Can you work these out from the model? Positions are in its coordinate system, mm. A direction names the side the tool comes from. Give positions to 0.01 mm unless a question says otherwise; leave off trailing zeros. Loops run counter-clockwise (first coordinate to the right, second up) from the corner with the lowest first, then second, coordinate; pieces in that order, holes last. Notation, with made-up numbers: (44.5, 36) - (67.5, 36) arc R19 cw to (67.5, 69) - close; hole circle Ø3 at (71.25, 80). An arc over 180 degrees is marked (long way). Answer as a JSON object with one key per item and string values. Group by question number.
Item 1: Which directions (+Z, -Z, +X, -X, +Y, -Y) give clear straight access to the entire face, cutting with the end or side of a thin tool? Please do faces 4 (the flat face through (0, -20, -2)), 5 (the flat face through (-1, 6, 0)), 6 (the cylindrical face through (1.46, -1.61, 6.95)).
Item 2: Please list where these lines run through material, in increasing order: L1, parallel to Z at x = 0.75, y = -15; L2, parallel to X at y = 23.5, z = 2.25; L3, parallel to Y at x = 0.25, z = -0.5.
Item 3: Will these pins go through, and if not, where does the flat tip stop? pin 1 (0.5 mm diameter, centred on x = 1, z = -0.5, fed in from +Y); pin 2 (1.5 mm diameter, centred on x = -1, y = 13, fed in from +Z); pin 3 (3.5 mm diameter, centred on x = 0, y = 16.5, fed in from -Z).
Item 4: Thinking about a two-plate mould opening in Z: for faces 1 (the cylindrical face through (0.046, -13.283, 4.541)), 2 (the flat face through (-1, -8, 8)), 3 (the flat face through (2.4, -3, 4)), which applies, pulls with the +Z half, pulls with the -Z half, needs draft (parallel to the pull), parting line crosses it, or undercut?
Item 5: Suppose I cut it at A-A on y = -15. Write out the boundary of the cut face in (x, z), and give its area (3 significant figures).
from build123d import *

# Parameters (mm, degrees)
F0_W     = 6.6
F0_H     = 14
F1_DEPTH = 8
F2_DEPTH = 2
F3_R     = 1.8
F4_DEPTH = 6.6
F5_R     = 6
F6_R     = 0.6
F7_DEPTH = 6
F8_R     = 1


with BuildPart() as f1:
    # F0 (on Top) → F1 (new body)
    with BuildSketch(Plane.XY):
        with Locations((0, -22)):
            Rectangle(F0_W, F0_H)
        Polygon((-3.3, -15), (3.3, -15), (3.3, -6), (2.4, -6), (2.4, 1), (1.2, 1), (1.2, 8), (0, 8), (0, 15), (-1.2, 15), (-1.2, 22), (-2.4, 22), (-2.4, 29), (-3.3, 29), align=None)
    extrude(amount=F1_DEPTH)

    # F0 (on Top) → F2 (join)
    with BuildSketch(Plane.XY):
        with Locations((0, -22)):
            Rectangle(F0_W, F0_H)
    extrude(amount=-F2_DEPTH)

    # F3 (on face) → F4 (cut)
    with BuildSketch(Plane.YZ.offset(3.3)):
        with Locations((-15, 4)):
            Circle(F3_R)
    extrude(amount=-F4_DEPTH, mode=Mode.SUBTRACT)

    # F5
    f5_edges = [f1.edges().sort_by_distance(p)[0] for p in [
        (2.85, -6, 8),
        (1.8, 1, 8),
        (0.6, 8, 8),
        (-0.6, 15, 8),
        (-1.8, 22, 8),
        (-2.85, 29, 8),
    ]]
    fillet(f5_edges, radius=F5_R)

    # F6
    f6_edges = [f1.edges().sort_by_distance(p)[0] for p in [
        (-2.4, 27.242641, 6.242641),
        (-2.4, 29, 1),
        (3.3, -20.5, 8),
        (2.4, -9, 8),
        (2.4, -5.5, 8),
        (-2.4, 22.5, 8),
        (1.2, -2, 8),
        (-2.4, 19, 8),
        (1.2, 1.5, 8),
        (-1.2, 15.5, 8),
        (0, 5, 8),
        (-1.2, 12, 8),
        (0, 8.5, 8),
        (-1.2, 22, 1),
        (-1.2, 20.242641, 6.242641),
        (0, 15, 1),
        (0, 13.242641, 6.242641),
        (1.2, 8, 1),
        (1.2, 6.242641, 6.242641),
        (2.4, 1, 1),
        (2.4, -0.757359, 6.242641),
        (3.3, -6, 1),
        (3.3, -7.757359, 6.242641),
    ]]
    fillet(f6_edges, radius=F6_R)

    # F7 (add): a face of the model
    f7_faces = [f1.faces().sort_by_distance(p)[0] for p in [
        (0, -15, -1),
    ]]
    extrude(f7_faces, amount=F7_DEPTH)

    # F8
    f8_edges = [f1.edges().sort_by_distance(p)[0] for p in [
        (0, -9, -2),
    ]]
    fillet(f8_edges, radius=F8_R)


solid = f1.part
Worked out:
{
 "1": {"face 4": "-Z, +X, -X, +Y, -Y", "face 5": "-Z, +X, -X, +Y", "face 6": "+Z, +X, +Y"},
 "2": {"L1": "z = -2 to 2.2, 5.8 to 8", "L2": "x = -3.3 to -2.4", "L3": "y = -29 to -9"},
 "3": {"pin 1": "stops at y = -9", "pin 2": "stops at z = 8", "pin 3": "stops at z = 0"},
 "4": {"face 1": "undercut", "face 2": "pulls with the +Z half", "face 3": "needs draft"},
 "5": {"outline": "(-3.3, -2) - (3.3, -2) - (3.3, 2.2) - (-3.3, 2.2) - close; (-3.3, 5.8) - (3.3, 5.8) - (3.3, 7.4) arc R0.6 ccw to (2.7, 8) - (-3.3, 8) - close", "area": "42.2 mm2"}
}
